Geometry: final body of the model. Coordinates: model frame, mm. Round coordinates to 2 decimals unless told otherwise and drop trailing zeros. Loops run counter-clockwise (first coordinate to the right, second up) from the corner with the lowest first, then second, coordinate; pieces in that order, holes last. Notation, with made-up numbers: (47.5, 87) -> (72.5, 87) arc R15 ccw to (72.5, 114) -> close; hole circle Ø6 at (76, 80). An arc over 180 degrees is marked (long way). Answer in a Markdown table with one row per item.
```python
from build123d import *

# Parameters (mm, degrees)
F0_W     = 1500
F0_H     = 200
F1_DEPTH = 20
F2_W     = 100
F2_H     = 10
F3_DEPTH = 20.001
F5_DEPTH = 20.001
F6_W     = 10
F6_H     = 50
F7_DEPTH = 20.001


with BuildPart() as f1:
    # F0 (on Top) → F1 (new body)
    with BuildSketch(Plane.XY):
        Rectangle(F0_W, F0_H)
    extrude(amount=F1_DEPTH)

    # F2 (on face) → F3 (cut, through all)
    with BuildSketch(Plane.XY.offset(20)):
        with Locations((-600, 95)):
            Rectangle(F2_W, F2_H)
        with Locations((-600, -95)):
            Rectangle(F2_W, F2_H)
        with Locations((-400, 95)):
            Rectangle(F2_W, F2_H)
        with Locations((-400, -95)):
            Rectangle(F2_W, F2_H)
        with Locations((-200, 95)):
            Rectangle(F2_W, F2_H)
        with Locations((-200, -95)):
            Rectangle(F2_W, F2_H)
        with Locations((0, 95)):
            Rectangle(F2_W, F2_H)
        with Locations((0, -95)):
            Rectangle(F2_W, F2_H)
        with Locations((200, 95)):
            Rectangle(F2_W, F2_H)
        with Locations((200, -95)):
            Rectangle(F2_W, F2_H)
        with Locations((400, 95)):
            Rectangle(F2_W, F2_H)
        with Locations((400, -95)):
            Rectangle(F2_W, F2_H)
        with Locations((600, 95)):
            Rectangle(F2_W, F2_H)
        with Locations((600, -95)):
            Rectangle(F2_W, F2_H)
    extrude(amount=-F3_DEPTH, mode=Mode.SUBTRACT)

    # F4 (on face) → F5 (cut, through all)
    with BuildSketch(Plane.XY.offset(20)):
        Polygon((-695, 50), (-705, 50), (-705, 5), (-750, 5), (-750, -5), (-705, -5), (-705, -50), (-695, -50), (-695, -5), (-650, -5), (-650, 5), (-695, 5), align=None)
        Polygon((-495, -50), (-495, -5), (-450, -5), (-450, 5), (-495, 5), (-495, 50), (-505, 50), (-505, 5), (-550, 5), (-550, -5), (-505, -5), (-505, -50), align=None)
        Polygon((-295, -50), (-295, -5), (-250, -5), (-250, 5), (-295, 5), (-295, 50), (-305, 50), (-305, 5), (-350, 5), (-350, -5), (-305, -5), (-305, -50), align=None)
        Polygon((-95, -50), (-95, -5), (-50, -5), (-50, 5), (-95, 5), (-95, 50), (-105, 50), (-105, 5), (-150, 5), (-150, -5), (-105, -5), (-105, -50), align=None)
        Polygon((105, -50), (105, -5), (150, -5), (150, 5), (105, 5), (105, 50), (95, 50), (95, 5), (50, 5), (50, -5), (95, -5), (95, -50), align=None)
        Polygon((305, -50), (305, -5), (350, -5), (350, 5), (305, 5), (305, 50), (295, 50), (295, 5), (250, 5), (250, -5), (295, -5), (295, -50), align=None)
        Polygon((505, -50), (505, -5), (550, -5), (550, 5), (505, 5), (505, 50), (495, 50), (495, 5), (450, 5), (450, -5), (495, -5), (495, -50), align=None)
        Polygon((705, -50), (705, -5), (750, -5), (750, 5), (705, 5), (705, 50), (695, 50), (695, 5), (650, 5), (650, -5), (695, -5), (695, -50), align=None)
    extrude(amount=-F5_DEPTH, mode=Mode.SUBTRACT)

    # F6 (on face) → F7 (cut, through all)
    with BuildSketch(Plane.XY.offset(20)):
        with Locations((-745, 75)):
            Rectangle(F6_W, F6_H)
        with Locations((-745, -75)):
            Rectangle(F6_W, F6_H)
        with Locations((745, 75)):
            Rectangle(F6_W, F6_H)
        with Locations((745, -75)):
            Rectangle(F6_W, F6_H)
    extrude(amount=-F7_DEPTH, mode=Mode.SUBTRACT)


solid = f1.part
```
Item 1: Cut plane C-C (x = 166). Output: boundary loops of the cut face in (y, z).
Answer:
| item | result |
|---|---|
| outline | (-90, 0) -> (90, 0) -> (90, 20) -> (-90, 20) -> close |
Item 2: Cut plane A-A (x = 482). Output: boundary loops of the cut face in (y, z), then the cut area to 3 significant figures.
Answer:
| item | result |
|---|---|
| outline | (-100, 0) -> (-5, 0) -> (-5, 20) -> (-100, 20) -> close; (5, 0) -> (100, 0) -> (100, 20) -> (5, 20) -> close |
| area | 3,800 mm² |
Item 3: Line query: probe 1 along Y at (x, z) = (107, 13.5); probe 2 along Y at (x, z) = (643.5, 1.5); probe 3 along X at (y, z) = (-51.5, 10.75). Output: solid intervals per line, ascending. Write a range as [from, to].
Answer:
| item | result |
|---|---|
| probe 1 | y = [-100, -5], [5, 100] |
| probe 2 | y = [-90, 90] |
| probe 3 | x = [-740, 740] |
Item 4: Pin query (flat end, axial travel): pin 1 Ø5 at (y, z) = (-96, 7) entering from -X; pin 2 Ø8 at (y, z) = (94.5, 13.5) entering from +X; pin 3 Ø6 at (x, z) = (-373.5, 9.5) entering from -Y. Return the tip coordinate at first contact, or that it passes through.
Answer:
| item | result |
|---|---|
| pin 1 | stops at x = -740 |
| pin 2 | stops at x = 740 |
| pin 3 | stops at y = -90 |
Item 5: Cut plane B-B (z = 3.25). Count the separate pieces of the cut face and the enclosed holes in it, then the cut area to 3 significant figures.
Answer:
| item | result |
|---|---|
| separate pieces | 1 |
| enclosed holes | 6 |
| area | 269,000 mm² |
